from build123d import *

# Parameters (mm, degrees)
SKETCH1_R           = 6.35
BOSS_EXTRUDE1_DEPTH = 152.4
SKETCH3_W           = 19.05
SKETCH3_H           = 12.7
CUT_EXTRUDE1_DEPTH  = 3.175
SKETCH4_W           = 19.05
SKETCH4_H           = 12.7
CUT_EXTRUDE2_DEPTH  = 3.175


with BuildPart() as part:
    # Sketch1 → Boss-Extrude1 (new body, symmetric)
    with BuildSketch(Plane(origin=(0, 0, 0), x_dir=(0, 0, -1), z_dir=(1, 0, 0))):
        Circle(SKETCH1_R)
    extrude(amount=BOSS_EXTRUDE1_DEPTH, both=True)

    # Sketch3 → Cut-Extrude1 (cut)
    with BuildSketch(Plane(origin=(0, 6.35, 0), x_dir=(1, 0, 0), z_dir=(0, 1, 0))):
        with Locations((130.175, 0)):
            Rectangle(SKETCH3_W, SKETCH3_H)
    extrude(amount=-CUT_EXTRUDE1_DEPTH, mode=Mode.SUBTRACT)

    # Sketch4 → Cut-Extrude2 (cut)
    with BuildSketch(Plane(origin=(0, 4.490128061, -4.490128061), x_dir=(1, 0, 0), z_dir=(0, -0.707106781, 0.707106781))):
        with Locations((-130.175, 0)):
            Rectangle(SKETCH4_W, SKETCH4_H)
    extrude(amount=CUT_EXTRUDE2_DEPTH, mode=Mode.SUBTRACT)


solid = part.part
Model file for the job. Use its own axes, mm. A direction names the side the tool comes from. Give positions to 0.01 mm unless a question says otherwise; leave off trailing zeros. Loops run counter-clockwise (first coordinate to the right, second up) from the corner with the lowest first, then second, coordinate; pieces in that order, holes last.
Item 1: Which spindle directions (+Z, -Z, +X, -X, +Y, -Y) get a long thin tool onto all of the face, cutting with end or side? Do faces 1 (the face through (130, 3.175, 0)), 2 (the face through (-120.65, 3, -3)), 3 (the face through (-152.4, 0, 0)). Say none if no direction does.
Check values:
face 1: +Z, -Z, +Y
face 2: -Z, +Y
face 3: +Z, -Z, -X, +Y, -Y
Item 2: Mould opens along X. For faces 4 (the face through (-139.7, 3, -3)), 5 (the face through (2.13, -6.2, 1.38)), 6 (the face through (152.4, 0, 0)) say: +X half, -X half, draft (parallel to the pull), parting line (faces both ways), or undercut.
Check values:
face 4: undercut
face 5: draft
face 6: +X half
Item 3: Slice it at B-B (x = 32.5). Write the cut outline in (y, z), plus the area to 3 significant figures.
Check values:
outline: circle Ø12.7 at (0, 0)
area: 127 mm2
Item 4: Drop flat-ended pins along their axis: P1, Ø5, axis at x = 26.5, z = 4.5, coming from the -Y side; P2, Ø5, axis at x = 49.5, z = -3.5, coming from the +Y side. Give the stop position or say it passes through.
Check values:
P1: stops at y = -6.03
P2: stops at y = 6.27
Item 5: Slice it at A-A (z = -2). Write the cut outline in (x, y) (3 decimals), plus the area to 3 significant figures.
Check values:
outline: (-152.4, -6.027) - (152.4, -6.027) - (152.4, 6.027) - (139.7, 6.027) - (139.7, 3.175) - (120.65, 3.175) - (120.65, 6.027) - (-120.65, 6.027) - (-120.65, 2.49) - (-139.7, 2.49) - (-139.7, 6.027) - (-152.4, 6.027) - close
area: 3,550 mm2
Item 6: Drill centre lines: line 1 along X through (y, z) = (4.5, 0.75); line 2 along Z through (x, y) = (113, 3.25); line 3 along Z through (x, y) = (-39.5, 1.5). Where is each one in solid material? Low to high.
Check values:
line 1: x = -152.4 to 120.65, 139.7 to 152.4
line 2: z = -5.46 to 5.46
line 3: z = -6.17 to 6.17
Item 7: Slice it at C-C (y = -4.25). Write the cut outline in (x, z).
Check values:
outline: (-152.4, -4.72) - (152.4, -4.72) - (152.4, 4.72) - (-152.4, 4.72) - close
